from build123d import *

# Parameters (mm, degrees)
SKETCH1_W                       = 100
SKETCH1_H                       = 100
BOSS_EXTRUDE1_DEPTH             = 700
FILLET1_R                       = 50
SKETCH2_R                       = 31
CUT_EXTRUDE1_DEPTH              = 100
F_5_0MM_DOWEL_HOLE1_D           = 5
F_5_0MM_DOWEL_HOLE1_CSINK_D     = 5.05
F_5_0MM_DOWEL_HOLE1_CSINK_ANGLE = 90
BOSS_EXTRUDE2_DEPTH             = 29.4
BOSS_EXTRUDE2_DEPTH_BACK        = 29.4
SKETCH6_R                       = 31
SKETCH6_R_2                     = 12.5


with BuildPart() as part:
    # Sketch1 → Boss-Extrude1 (new body)
    with BuildSketch(Plane(origin=(0, 0, 0), x_dir=(0, 1, 0), z_dir=(0, 0, 1))):
        Rectangle(SKETCH1_W, SKETCH1_H)
    extrude(amount=-BOSS_EXTRUDE1_DEPTH)

    # Fillet1
    fillet1_edges = [part.edges().sort_by_distance(p)[0] for p in [
        (0, -50, -700),
        (0, 50, -700),
    ]]
    fillet(fillet1_edges, radius=FILLET1_R - 0.0001)  # a hair under: the kernel refuses the full size

    # Sketch2 → Cut-Extrude1 (cut)
    with BuildSketch(Plane.YZ.offset(50)):
        with Locations((0, -650)):
            Circle(SKETCH2_R)
    extrude(amount=-CUT_EXTRUDE1_DEPTH, mode=Mode.SUBTRACT)

    # Ø5.0mm Dowel Hole1 (through all)
    with Locations(Plane.XZ.offset(50)):
        with Locations((0, -25)):
            f_5_0mm_dowel_hole1 = CounterSinkHole(F_5_0MM_DOWEL_HOLE1_D / 2, F_5_0MM_DOWEL_HOLE1_CSINK_D / 2, counter_sink_angle=F_5_0MM_DOWEL_HOLE1_CSINK_ANGLE)

    # Mirror1: Ø5.0mm Dowel Hole1 across plane
    add(f_5_0mm_dowel_hole1.mirror(Plane.ZX), mode=Mode.SUBTRACT)

    # Sketch6 → Boss-Extrude2 (add, two sides: drawn at the far end of the back side and taken through both)
    with BuildSketch(Plane.YZ.offset(-BOSS_EXTRUDE2_DEPTH_BACK)):
        with Locations(Location((0, -650, 0), (0, 0, 270))):
            Circle(SKETCH6_R)
        with Locations(Location((0, -650, 0), (0, 0, 270))):
            Circle(SKETCH6_R_2, mode=Mode.SUBTRACT)
    extrude(amount=BOSS_EXTRUDE2_DEPTH + BOSS_EXTRUDE2_DEPTH_BACK)


solid = part.part
For this review, take the finished solid that the model builds, in its own axes (mm). A direction names the side the tool comes from. Give positions to 0.01 mm unless a question says otherwise; leave off trailing zeros. Loops run counter-clockwise (first coordinate to the right, second up) from the corner with the lowest first, then second, coordinate; pieces in that order, holes last. Notation, with made-up numbers: M 41,81.25 L 75,81.25 A22 ccw 75,109.25 Z; hole C 17,-22.75 d5. An arc over 180 degrees is marked long. Put each result on its own line as item: value. Start each with the question number.
(1) Add section C-C, the plane y = 21. Write out the cut boundary in (x, z).
(2) Add section B-B, the plane y = -43.5. Write out the cut boundary in (x, z).
(3) The part is to be moulded in two halves that separate along Z. For faces 4 (the cylindrical face through (-39.556, 14.305, -677.502)), 5 (the flat face through (-50, -1, -345)), 6 (the cylindrical face through (-0.7, -35.742, -684.964)), say which applies: +Z half, -Z half, draft (parallel to the pull), parting line (faces both ways), or undercut.
(4) Machinability: for faces 1 (the flat face through (-1, -1, 0)), 2 (the flat face through (-29.4, -13, -650)), 3 (the cylindrical face through (39.844, 14.305, -677.502)), which of the approach directions +Z, -Z, +X, -X, +Y, -Y give a long, thin tool a straight path to every point of the face, cutting with its end or side? Answer none if there is none.
(5) Wall thickness on L1, parallel to X at y = 22, z = -25; L2, parallel to Y at x = -38, z = -650; L3, parallel to Z at x = 44.5, y = 0: over which ranges is each line inside the solid? List them lowest first.
Result:
1. outline: M -50,-695.38 L 50,-695.38 L 50,-672.8 L 29.4,-672.8 L 29.4,-627.2 L 50,-627.2 L 50,0 L -50,0 L -50,-627.2 L -29.4,-627.2 L -29.4,-672.8 L -50,-672.8 Z; hole C 0,-25 d5
2. outline: M -50,-674.65 L 50,-674.65 L 50,0 L -50,0 Z; hole C 0,-25 d5
3. face 4: undercut
3. face 5: draft
3. face 6: -Z half
4. face 1: +Z, +X, -X, +Y, -Y
4. face 2: -X
4. face 3: +X
5. L1: x = -50 to -2.5, 2.5 to 50
5. L2: y = -50 to -31, 31 to 50
5. L3: z = -700 to -681, -619 to 0
